Build history of the part. All positions in model axes, mm. A direction names the side the tool comes from. Coordinates: 2 decimals unless noted, no trailing zeros. Write each question's results on one line, items separated by ' | '. Start each with the question number.
Q1. Drill centre lines: line 1 (X direction, y = 0, z = 5.25); line 2 (Y direction, x = 0, z = 5); line 3 (Y direction, x = -5.5, z = 4.25). Where is each one in solid material? Low to high.
Q2. Tool access for faces 1 (the face through (4.542, -18.926, 4.517)), 2 (the face through (4.536, 18.9, 4.517)), 3 (the face through (9.11, -14.3, 9.42)): list every direction of +Z, -Z, +X, -X, +Y, -Y with a clear straight run to the whole face (end or side of a thin tool).
Q3. Two-plate mould, pull along X, no slides. Class faces 4 (the face through (-11, 11, 3.277)), 5 (the face through (-19, 0, 6.985)), 6 (the face through (9.3, -14.6, 8.5)): released by +X, released by -X, zero draft, split by the parting line, or undercut.
Q4. Drop flat-ended pins along their axis: pin 1 Ø5 at (x, z) = (9, 7.5) entering from -Y; pin 2 Ø1.5 at (x, z) = (3, 4) entering from +Y; pin 3 Ø3 at (x, z) = (-9, 7.5) entering from +Y. Give the stop position or say it passes through.
from build123d import *

# Parameters (mm, degrees)
F2_R     = 0.79502
F4_DEPTH = 9.653
F5_R     = 0.79502


with BuildPart() as f1:
    # F0 (on Front) → F1 (revolve)
    with BuildSketch(Plane.XZ):
        Polygon((16.9545, 9.652), (15.0368, 9.652), (15.0368, 3.2766), (16.9672, 3.2766), (16.9672, 0), (18.5547, 0), (18.5547, 1.3208), (20.3962, 1.3208), (20.3962, 6.985), (18.82648, 6.985), (16.9545, 8.85698), align=None)
    revolve(axis=Axis((0, 0, 4.540607), (0, 0, -1)))

    # F2
    f2_edges = [f1.edges().sort_by_distance(p)[0] for p in [
        (-16.9672, 0, 3.2766),
    ]]
    fillet(f2_edges, radius=F2_R)

    # F3 (on face) → F4 (cut, through all)
    with BuildSketch(Plane.XY.offset(9.652)):
        with BuildLine():
            Line((-4.75958, 19.833088), (-4.318, 17.993032))
            ThreePointArc((-4.318, 17.993032), (0, 18.5039), (4.318, 17.993032))
            Line((4.318, 17.993032), (4.75958, 19.833088))
            ThreePointArc((4.75958, 19.833088), (0, 20.3962), (-4.75958, 19.833088))
        make_face()
        with BuildLine():
            ThreePointArc((4.318, -17.993032), (0, -18.5039), (-4.318, -17.993032))
            Line((-4.318, -17.993032), (-4.75958, -19.833088))
            ThreePointArc((-4.75958, -19.833088), (0, -20.3962), (4.75958, -19.833088))
            Line((4.75958, -19.833088), (4.318, -17.993032))
        make_face()
    extrude(amount=-F4_DEPTH, mode=Mode.SUBTRACT)

    # F5
    f5_edges = [f1.edges().sort_by_distance(p)[0] for p in [
        (-16.9545, 0, 8.85698),
    ]]
    fillet(f5_edges, radius=F5_R)


solid = f1.part
Returned:
1) line 1: x = -20.4 to -15.04, 15.04 to 20.4 | line 2: y = -18.5 to -15.04, 15.04 to 18.5 | line 3: y = -19.64 to -13.99, 13.99 to 19.64
2) face 1: +Z, -Z, -Y | face 2: +Z, -Z, +Y | face 3: +Z
3) face 4: undercut | face 5: zero draft | face 6: split by the parting line
4) pin 1: stops at y = -19.31 | pin 2: stops at y = 18.37 | pin 3: stops at y = 18.93
